```python
from build123d import *

# Parameters (mm, degrees)
SKETCH_1_R      = 1.5
EXTRUDE_1_DEPTH = 2


with BuildPart() as part:
    # 草图1 → 凸台-拉伸1 (new body)
    # profile 1 of 2: a face of its own
    with BuildSketch(Plane(origin=(0, 0, 0), x_dir=(1, 0, 0), z_dir=(0, 1, 0))):
        with BuildLine():
            Line((6, 50), (4, 50))
            ThreePointArc((4, 50), (1.171572875, 48.828427125), (0, 46))
            Line((0, 46), (0, 0))
            Line((0, 0), (120, 0))
            Line((120, 0), (120, 15))
            ThreePointArc((120, 15), (121.464466094, 18.535533906), (125, 20))
            Line((125, 20), (135, 20))
            ThreePointArc((135, 20), (138.535533906, 18.535533906), (140, 15))
            Line((140, 15), (140, 0))
            Line((140, 0), (320, 0))
            Line((320, 0), (320, 46))
            ThreePointArc((320, 46), (318.828427125, 48.828427125), (316, 50))
            Line((316, 50), (310, 50))
            ThreePointArc((310, 50), (308.585786438, 49.414213562), (308, 48))
            Line((308, 48), (308, 37))
            ThreePointArc((308, 37), (306.535533906, 33.464466094), (303, 32))
            Line((303, 32), (239, 32))
            ThreePointArc((239, 32), (235.464466094, 33.464466094), (234, 37))
            Line((234, 37), (234, 48))
            ThreePointArc((234, 48), (233.414213562, 49.414213562), (232, 50))
            Line((232, 50), (94, 50))
            ThreePointArc((94, 50), (92.585786438, 49.414213562), (92, 48))
            Line((92, 48), (92, 37))
            ThreePointArc((92, 37), (90.535533906, 33.464466094), (87, 32))
            Line((87, 32), (23, 32))
            ThreePointArc((23, 32), (19.464466094, 33.464466094), (18, 37))
            Line((18, 37), (18, 48))
            ThreePointArc((18, 48), (17.414213562, 49.414213562), (16, 50))
            Line((16, 50), (6, 50))
        make_face()
        with Locations(Location((4.503217652, 40, 0), (0, 0, 270))):
            Circle(SKETCH_1_R, mode=Mode.SUBTRACT)
        with Locations(Location((98, 40, 0), (0, 0, 270))):
            Circle(SKETCH_1_R, mode=Mode.SUBTRACT)
        with Locations(Location((222, 40, 0), (0, 0, 270))):
            Circle(SKETCH_1_R, mode=Mode.SUBTRACT)
        with Locations(Location((314, 40, 0), (0, 0, 270))):
            Circle(SKETCH_1_R, mode=Mode.SUBTRACT)
    # profile 2 of 2: a face of its own
    with BuildSketch(Plane(origin=(0, 0, 0), x_dir=(1, 0, 0), z_dir=(0, 1, 0))):
        with BuildLine():
            Line((120, 0), (0, 0))
            Line((0, 0), (0, -46))
            ThreePointArc((0, -46), (1.171572875, -48.828427125), (4, -50))
            Line((4, -50), (6, -50))
            Line((6, -50), (16, -50))
            ThreePointArc((16, -50), (17.414213562, -49.414213562), (18, -48))
            Line((18, -48), (18, -37))
            ThreePointArc((18, -37), (19.464466094, -33.464466094), (23, -32))
            Line((23, -32), (87, -32))
            ThreePointArc((87, -32), (90.535533906, -33.464466094), (92, -37))
            Line((92, -37), (92, -48))
            ThreePointArc((92, -48), (92.585786438, -49.414213562), (94, -50))
            Line((94, -50), (232, -50))
            ThreePointArc((232, -50), (233.414213562, -49.414213562), (234, -48))
            Line((234, -48), (234, -37))
            ThreePointArc((234, -37), (235.464466094, -33.464466094), (239, -32))
            Line((239, -32), (303, -32))
            ThreePointArc((303, -32), (306.535533906, -33.464466094), (308, -37))
            Line((308, -37), (308, -48))
            ThreePointArc((308, -48), (308.585786438, -49.414213562), (310, -50))
            Line((310, -50), (316, -50))
            ThreePointArc((316, -50), (318.828427125, -48.828427125), (320, -46))
            Line((320, -46), (320, 0))
            Line((320, 0), (140, 0))
            Line((140, 0), (140, -15))
            ThreePointArc((140, -15), (138.535533906, -18.535533906), (135, -20))
            Line((135, -20), (125, -20))
            ThreePointArc((125, -20), (121.464466094, -18.535533906), (120, -15))
            Line((120, -15), (120, 0))
        make_face()
        with Locations(Location((4.503217652, -40, 0), (0, 0, 270))):
            Circle(SKETCH_1_R, mode=Mode.SUBTRACT)
        with Locations(Location((98, -40, 0), (0, 0, 270))):
            Circle(SKETCH_1_R, mode=Mode.SUBTRACT)
        with Locations(Location((222, -40, 0), (0, 0, 270))):
            Circle(SKETCH_1_R, mode=Mode.SUBTRACT)
        with Locations(Location((314, -40, 0), (0, 0, 270))):
            Circle(SKETCH_1_R, mode=Mode.SUBTRACT)
    extrude(amount=EXTRUDE_1_DEPTH)


solid = part.part
```
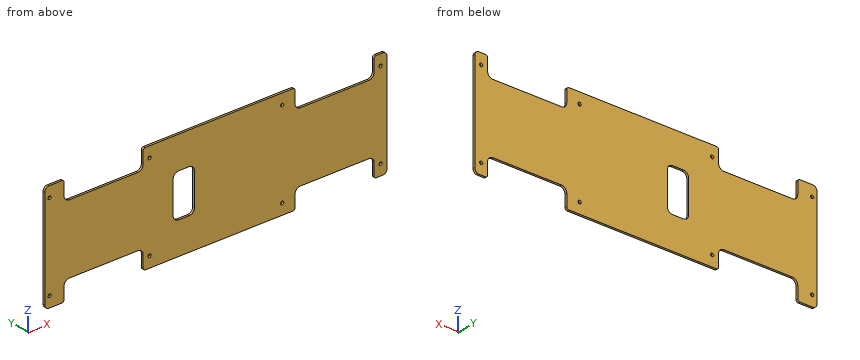
Model file for the job. Use its own axes, mm. Give positions to 0.01 mm unless a question says otherwise; leave off trailing zeros. Loops run counter-clockwise (first coordinate to the right, second up) from the corner with the lowest first, then second, coordinate; pieces in that order, holes last. Notation, with made-up numbers: M 67.25,32 L 111.25,32 A5 cw 111.25,37 Z; hole C 34,11 d8. An arc over 180 degrees is marked long. Use one line per item in the form item = value.
Item 1: Slice it at A-A on x = 269. List the corners of the cut face in (y, z), and give its area (3 significant figures).
Filled in:
outline = M 0,-32 L 2,-32 L 2,32 L 0,32 Z
area = 128 mm^2
Item 2: Slice it at B-B on y = 1.4. Give the number of separate pieces and of enclosed holes in the cut face, and give its area (3 significant figures).
Filled in:
separate_pieces = 1
enclosed_holes = 9
area = 25,900 mm^2
Item 3: Drill centre lines: L1, parallel to Z at x = 314, y = 1.2; L2, parallel to X at y = 1.35, z = 0; L3, parallel to Z at x = 261, y = 0.2. Where is each one in solid material? Low to high.
Filled in:
L1 = -50 to -41.5, -38.5 to 38.5, 41.5 to 50
L2 = 0 to 120, 140 to 320
L3 = -32 to 32
Item 4: Flat gauge pins, fed straight in: pin 1 Ø0.6 at (x, y) = (283, 1.5) entering from +Z; pin 2 Ø3.5 at (x, z) = (314, 40) entering from +Y; pin 3 Ø0.6 at (x, y) = (43.5, 1.5) entering from -Z. Where does each tip first touch, or does it go through?
Filled in:
pin_1 = 32
pin_2 = 2
pin_3 = -32
